Can you work these out from the model? Positions are in its coordinate system, mm. A direction names the side the tool comes from. Give positions to 0.01 mm unless a question says otherwise; leave off trailing zeros. Order: outer loops, then holes, each group sorted by start corner. A loop starts at its lowest first (then second) coordinate and runs counter-clockwise, first axis right, second up. Notation, with made-up numbers: (-20.5, 60.25) - (11.5, 60.25) arc R14 cw to (11.5, 69.25) - close; hole circle Ø4 at (34.5, 22). An arc over 180 degrees is marked (long way). Answer as a JSON object with one key per item and string values.
```python
from build123d import *

# Parameters (mm, degrees)
SKETCH_1_W               = 25
SKETCH_1_H               = 55
EXTRUDE_1_DEPTH          = 3
SKETCH_7_W               = 10
SKETCH_7_H               = 10
EXTRUDE_2_DEPTH          = 20
HOLE_WIZARD_2_D          = 10
SKETCH_4_W               = 1.75
SKETCH_4_H               = 3
HOLE_WIZARD_1_AT_2_COUNT = 2
HOLE_WIZARD_1_AT_2_PITCH = 15
HOLE_WIZARD_1_AT_3_COUNT = 2
HOLE_WIZARD_1_AT_3_PITCH = 47.434164903
HOLE_WIZARD_1_AT_4_COUNT = 2
HOLE_WIZARD_1_AT_4_PITCH = 45
HOLE_WIZARD_3_D          = 3.5


with BuildPart() as part:
    # 草图1 → 凸台-拉伸1 (new body)
    with BuildSketch(Plane(origin=(0, 0, 0), x_dir=(1, 0, 0), z_dir=(0, 1, 0))):
        Rectangle(SKETCH_1_W, SKETCH_1_H)
    extrude(amount=EXTRUDE_1_DEPTH)

    # 草图7 → 凸台-拉伸2 (add)
    with BuildSketch(Plane(origin=(0, 3, 0), x_dir=(1, 0, 0), z_dir=(0, 1, 0))):
        with Locations((-7.5, 22.5)):
            Rectangle(SKETCH_7_W, SKETCH_7_H)
        with Locations((7.5, 22.5)):
            Rectangle(SKETCH_7_W, SKETCH_7_H)
        with Locations((7.5, -22.5)):
            Rectangle(SKETCH_7_W, SKETCH_7_H)
        with Locations((-7.5, -22.5)):
            Rectangle(SKETCH_7_W, SKETCH_7_H)
    extrude(amount=EXTRUDE_2_DEPTH)

    # 孔2 (through all)
    with Locations(Plane(origin=(0, 3, 0), x_dir=(1, 0, 0), z_dir=(0, 1, 0))):
        with Locations((0, -2)):
            Hole(HOLE_WIZARD_2_D / 2)

    # 草图4 → 孔1 (revolve, cut)
    with BuildSketch(Plane(origin=(-7.5, 3, -22.5), x_dir=(0, 0, 1), z_dir=(1, 0, 0))):
        with Locations((0.875, 1.5)):
            Rectangle(SKETCH_4_W, SKETCH_4_H)
    hole_wizard_1 = revolve(axis=Axis((-7.5, -107, -22.5), (0, 1, 0)), mode=Mode.SUBTRACT)

    # 孔1 at 2: 孔1 ×2
    with Locations(*[(i * HOLE_WIZARD_1_AT_2_PITCH, 0, 0) for i in range(1, HOLE_WIZARD_1_AT_2_COUNT)]):
        add(hole_wizard_1, mode=Mode.SUBTRACT)

    # 孔1 at 3: 孔1 ×2
    with Locations(*[Vector(0.3162277660168381, 0, 0.9486832980505139) * (i * HOLE_WIZARD_1_AT_3_PITCH) for i in range(1, HOLE_WIZARD_1_AT_3_COUNT)]):
        add(hole_wizard_1, mode=Mode.SUBTRACT)

    # 孔1 at 4: 孔1 ×2
    with Locations(*[(0, 0, i * HOLE_WIZARD_1_AT_4_PITCH) for i in range(1, HOLE_WIZARD_1_AT_4_COUNT)]):
        add(hole_wizard_1, mode=Mode.SUBTRACT)

    # 孔3 (through all)
    with Locations(Plane(origin=(0, 0, 0), x_dir=(-1, 0, 0), z_dir=(0, -1, 0))):
        with Locations((7.5, 22.5), (-7.5, 22.5), (-7.5, -22.5), (7.5, -22.5)):
            Hole(HOLE_WIZARD_3_D / 2)


solid = part.part
```
Q1. If we section it at D-D, the plane z = 21.5: Please give me the cut outline in (x, y), then the cut area to 3 significant figures.
Recorded:
{"outline": "(-12.5, 0) - (-8.94, 0) - (-8.94, 23) - (-12.5, 23) - close; (-6.06, 0) - (6.06, 0) - (6.06, 23) - (2.5, 23) - (2.5, 3) - (-2.5, 3) - (-2.5, 23) - (-6.06, 23) - close; (8.94, 0) - (12.5, 0) - (12.5, 23) - (8.94, 23) - close", "area": "343 mm^2"}
Q2. I need wall thicknesses on L1, parallel to Z at x = 7.5, y = 16.25; L2, parallel to X at y = 15.75, z = 22.5; L3, parallel to Z at x = -5, y = 10.25. Which ranges of each line are inside material? Lowest first, please.
Recorded:
{"L1": "z = -27.5 to -24.25, -20.75 to -17.5, 17.5 to 20.75, 24.25 to 27.5", "L2": "x = -12.5 to -9.25, -5.75 to -2.5, 2.5 to 5.75, 9.25 to 12.5", "L3": "z = -27.5 to -17.5, 17.5 to 27.5"}
Q3. If we section it at B-B, the plane x = 0: Please give me the cut outline in (y, z), then the cut area to 3 significant figures.
Recorded:
{"outline": "(0, -27.5) - (3, -27.5) - (3, -3) - (0, -3) - close; (0, 7) - (3, 7) - (3, 27.5) - (0, 27.5) - close", "area": "135 mm^2"}
Q4. We'd pull the mould along X, two halves only. Please class faces 4 (the face through (2.5, 13, 23)), 5 (the face through (12.5, 1, 0)), 6 (the face through (7, 13, 17.5)), 7 (the face through (-2.5, 13, 23)): released by +X, released by -X, zero draft, split by the parting line, or undercut.
Recorded:
{"face 4": "undercut", "face 5": "released by +X", "face 6": "zero draft", "face 7": "undercut"}
Q5. If we section it at C-C, the plane z = 2: Please give me the cut outline in (x, y), then the cut area to 3 significant figures.
Recorded:
{"outline": "(-12.5, 0) - (-5, 0) - (-5, 3) - (-12.5, 3) - close; (5, 0) - (12.5, 0) - (12.5, 3) - (5, 3) - close", "area": "45.0 mm^2"}
Q6. If we section it at A-A, the plane y = 8.5: Please give me the cut outline in (x, z).
Recorded:
{"outline": "(-12.5, -27.5) - (-2.5, -27.5) - (-2.5, -17.5) - (-12.5, -17.5) - close; (-12.5, 17.5) - (-2.5, 17.5) - (-2.5, 27.5) - (-12.5, 27.5) - close; (2.5, -27.5) - (12.5, -27.5) - (12.5, -17.5) - (2.5, -17.5) - close; (2.5, 17.5) - (12.5, 17.5) - (12.5, 27.5) - (2.5, 27.5) - close; hole circle Ø3.5 at (-7.5, -22.5); hole circle Ø3.5 at (-7.5, 22.5); hole circle Ø3.5 at (7.5, -22.5); hole circle Ø3.5 at (7.5, 22.5)"}
Q7. Which directions (+Z, -Z, +X, -X, +Y, -Y) give clear straight access to the entire face, cutting with the end or side of a thin tool? Please do faces 1 (the face through (-8, 13, -17.5)), 2 (the face through (1.08, 1.48, 6.88)), 3 (the face through (-2.5, 13, -22)).
Recorded:
{"face 1": "+X, -X, +Y", "face 2": "+Y, -Y", "face 3": "+Z, -Z, +Y"}
Q8. I'm going to push flat-ended pins straight in: pin 1 Ø10 at (y, z) = (6.5, 9.5) entering from +X; pin 2 Ø11.5 at (x, z) = (0, 2) entering from +Y. Where does each tip first touch, or does it pass through?
Recorded:
{"pin 1": "stops at x = 12.5", "pin 2": "stops at y = 3"}
